Autodesk Inventor part; units mm, degrees
ref_plane "YZ Plane" through (0, 0, 0) normal (1, 0, 0) x (0, 1, 0)
ref_plane "XZ Plane" through (0, 0, 0) normal (0, 1, 0) x (-1, 0, 0)
ref_plane "XY Plane" through (0, 0, 0) normal (0, 0, 1) x (1, 0, 0)
sketch "Sketch1" plane through (0, 0, 0) normal (0, 0, 1) x (1, 0, 0)
  circle A0 centre (0, 0) radius 27.9
  line L0 (-24, 12.5) -> (24, 12.5)
  line L1 (24, 12.5) -> (24, -12.5)
  line L2 (24, -12.5) -> (-24, -12.5)
  line L3 (-24, -12.5) -> (-24, 12.5)
  dimension "d0" = 55.8
  dimension "d1" = 48
  dimension "d2" = 24
  dimension "d3" = 25
  dimension "d4" = 12.5
extrude "Extrusion1" add sketch "Sketch1" along normal mid plane 15
sketch "Sketch2" plane through (0, 0, 7.5) normal (0, 0, 1) x (1, 0, 0)
  circle A0 centre (0, 0) radius 27.9
  dimension "d10" = 55.8
extrude "Extrusion2" add sketch "Sketch2" against normal blind 5
fillet "Fillet1" radius 1 4 edges at (-24, 0, -7.5) (0, 12.5, -7.5) (0, -12.5, -7.5) (24, 0, -7.5)
properties part number "soporte base pila"
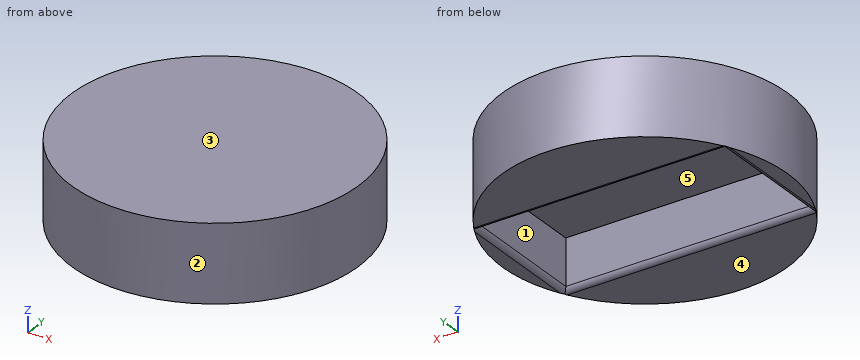
Here's how the part is built. I have some questions about the finished solid (model axes, mm). Face numbers are marked on the shaded views. A direction names the side the tool comes from. Coordinates: 2 decimals unless noted, no trailing zeros. Loops run counter-clockwise (first coordinate to the right, second up) from the corner with the lowest first, then second, coordinate; pieces in that order, holes last. Notation, with made-up numbers: (67.25, -13) - (106.25, -13) arc R8 ccw to (106.25, -6) - close; hole circle Ø4 at (75.5, -1). An arc over 180 degrees is marked (long way). Return JSON: item names as keys, results as strings. Group by question number.
Item 1: If we section it at A-A on y = 0: Write out the boundary of the cut face in (x, z), and give its area (3 significant figures).
Item 2: I need wall thicknesses on line 1 (Z direction, x = -18.5, y = 5); line 2 (Y direction, x = -0.5, z = -6.5); line 3 (Y direction, x = 11, z = -0.25). Which ranges of each line are inside material? Lowest first, please. Write a range as from..to.
Item 3: On a 3-axis mill with a long thin cutter (end or side, diameter ignored), from which of +Z, -Z, +X, -X, +Y, -Y can I reach the whole of each face in a straight line? I mean the marked faces 4 and 5. Say none if no direction works.
Item 4: Will these pins go through, and if not, where does the flat tip stop? P1, Ø6, axis at y = -5.5, z = -5.5, coming from the -X side; P2, Ø12.5, axis at x = 4, y = 5, coming from the -Z side; P3, Ø1, axis at y = 21, z = -2, coming from the +X side; P4, Ø4.5, axis at y = 2, z = -4, coming from the +X side.
Item 5: We'd pull the mould along Y, two halves only. Please class the marked faces 1, 2 and 3: +Y half, -Y half, draft (parallel to the pull), parting line (faces both ways), or undercut.
Item 6: If we section it at C-C on z = 1: Write out the boundary of the cut face in (x, y).
Item 7: If we section it at D-D on z = 4.5: Write out the boundary of the cut face in (x, y).
Item 8: If we section it at B-B on x = 0: Write out the boundary of the cut face in (y, z), and give its area (3 significant figures).
Calculated:
{
 "1": {"outline": "(-27.9, -7.5) - (-25, -7.5) arc R1 ccw to (-24, -6.5) - (-24, 2.5) - (24, 2.5) - (24, -6.5) arc R1 ccw to (25, -7.5) - (27.9, -7.5) - (27.9, 7.5) - (-27.9, 7.5) - close", "area": "357 mm^2"},
 "2": {"line 1": "z = 2.5..7.5", "line 2": "y = -27.9..-12.5, 12.5..27.9", "line 3": "y = -25.64..-12.5, 12.5..25.64"},
 "3": {"face 4": "-Z, +X, -X, +Y, -Y", "face 5": "-Z"},
 "4": {"P1": "stops at x = -27.79", "P2": "stops at z = 2.5", "P3": "stops at x = 18.93", "P4": "stops at x = 27.9"},
 "5": {"face 1": "undercut", "face 2": "parting line", "face 3": "draft"},
 "6": {"outline": "circle Ø55.8 at (0, 0); hole (-24, -12.5) - (24, -12.5) - (24, 12.5) - (-24, 12.5) - close"},
 "7": {"outline": "circle Ø55.8 at (0, 0)"},
 "8": {"outline": "(-27.9, -7.5) - (-13.5, -7.5) arc R1 ccw to (-12.5, -6.5) - (-12.5, 2.5) - (12.5, 2.5) - (12.5, -6.5) arc R1 ccw to (13.5, -7.5) - (27.9, -7.5) - (27.9, 7.5) - (-27.9, 7.5) - close", "area": "587 mm^2"}
}
